```python
from build123d import *

# Parameters (mm, degrees)
SKETCH4_R           = 3.5
SKETCH4_R_2         = 19.25
BOSS_EXTRUDE1_DEPTH = 1
SKETCH5_R           = 19.25
BOSS_EXTRUDE2_DEPTH = 5
SKETCH6_R           = 18.5
BOSS_EXTRUDE3_DEPTH = 2
CUT_EXTRUDE1_DEPTH  = 6
SKETCH8_W           = 1
SKETCH8_H           = 25
CUT_EXTRUDE2_DEPTH  = 6
BOSS_EXTRUDE4_START = 4
SKETCH9_W           = 20
SKETCH9_H           = 18
BOSS_EXTRUDE4_DEPTH = 4
SKETCH10_R          = 4
BOSS_EXTRUDE5_DEPTH = 22
SKETCH11_R          = 3.5
BOSS_EXTRUDE6_DEPTH = 4
SKETCH12_R          = 2.75
CUT_EXTRUDE3_DEPTH  = 2
SKETCH13_R          = 1.5
CUT_EXTRUDE4_DEPTH  = 7
SKETCH14_W          = 35.5
SKETCH14_H          = 26
BOSS_EXTRUDE7_DEPTH = 20
BOSS_EXTRUDE8_DEPTH = 9.5
SKETCH16_W          = 15.5
SKETCH16_H          = 5
CUT_EXTRUDE5_DEPTH  = 8.5
SKETCH17_R          = 2
CUT_EXTRUDE6_DEPTH  = 4


with BuildPart() as part:
    # Sketch4 → Boss-Extrude1 (new body)
    with BuildSketch(Plane(origin=(0, 0, 0), x_dir=(1, 0, 0), z_dir=(0, 1, 0))):
        with Locations((-17.75, -21.25)):
            Circle(SKETCH4_R)
        with BuildLine():
            ThreePointArc((3e-08, -19.25), (-13.611805493, -13.611805583), (-19.25, -9.7e-08))
            Line((-19.25, -9.7e-08), (-19.25, -13))
            Line((-19.25, -13), (-21.140562134, -20.381617358))
            ThreePointArc((-21.140562134, -20.381617358), (-17.312374287, -17.777467245), (-14.25, -21.25))
            ThreePointArc((-14.25, -21.25), (-14.66103595, -22.895691677), (-15.797600627, -24.154847102))
            Line((-15.797600627, -24.154847102), (-8.5, -19.25))
            Line((-8.5, -19.25), (3e-08, -19.25))
        make_face()
        Circle(SKETCH4_R_2)
        with BuildLine():
            Line((19.25, -13), (19.25, 0))
            ThreePointArc((19.25, 0), (13.611805548, -13.611805527), (3e-08, -19.25))
            Line((3e-08, -19.25), (8.5, -19.25))
            Line((8.5, -19.25), (15.797600627, -24.154847102))
            ThreePointArc((15.797600627, -24.154847102), (15.7309919, -18.391048043), (21.140562134, -20.381617358))
            Line((21.140562134, -20.381617358), (19.25, -13))
        make_face()
        with Locations((17.75, -21.25)):
            Circle(SKETCH4_R)
        with BuildLine():
            Line((8.5, 19.25), (0, 19.25))
            ThreePointArc((0, 19.25), (13.611805538, 13.611805538), (19.25, 0))
            Line((19.25, 0), (19.25, 13))
            Line((19.25, 13), (21.140562134, 20.381617358))
            ThreePointArc((21.140562134, 20.381617358), (15.7309919, 18.391048043), (15.797600627, 24.154847102))
            Line((15.797600627, 24.154847102), (8.5, 19.25))
        make_face()
        with Locations((17.75, 21.25)):
            Circle(SKETCH4_R)
        with BuildLine():
            Line((-8.5, 19.25), (-15.797600627, 24.154847102))
            ThreePointArc((-15.797600627, 24.154847102), (-14.66103595, 22.895691677), (-14.25, 21.25))
            ThreePointArc((-14.25, 21.25), (-17.312374287, 17.777467245), (-21.140562134, 20.381617358))
            Line((-21.140562134, 20.381617358), (-19.25, 13))
            Line((-19.25, 13), (-19.25, -9.7e-08))
            ThreePointArc((-19.25, -9.7e-08), (-13.611805572, 13.611805504), (0, 19.25))
            Line((0, 19.25), (-8.5, 19.25))
        make_face()
        with Locations((-17.75, 21.25)):
            Circle(SKETCH4_R)
    extrude(amount=BOSS_EXTRUDE1_DEPTH)

    # Sketch5 → Boss-Extrude2 (add)
    with BuildSketch(Plane(origin=(0, 1, 0), x_dir=(1, 0, 0), z_dir=(0, 1, 0))):
        with Locations(Location((0, 0, 0), (0, 0, 270))):
            Circle(SKETCH5_R)
    extrude(amount=BOSS_EXTRUDE2_DEPTH)

    # Sketch6 → Boss-Extrude3 (add)
    with BuildSketch(Plane(origin=(0, 6, 0), x_dir=(1, 0, 0), z_dir=(0, 1, 0))):
        with Locations(Location((0, 0, 0), (0, 0, 270))):
            Circle(SKETCH6_R)
    extrude(amount=BOSS_EXTRUDE3_DEPTH)

    # Sketch7 → Cut-Extrude1 (cut)
    with BuildSketch(Plane(origin=(0, 8, 0), x_dir=(1, 0, 0), z_dir=(0, 1, 0))):
        with BuildLine():
            Line((-11.5, 13), (11.5, 13))
            ThreePointArc((11.5, 13), (17.356554958, 0), (11.5, -13))
            Line((11.5, -13), (-11.5, -13))
            ThreePointArc((-11.5, -13), (-17.356554958, 0), (-11.5, 13))
        make_face()
    extrude(amount=-CUT_EXTRUDE1_DEPTH, mode=Mode.SUBTRACT)

    # Sketch8 → Cut-Extrude2 (cut)
    with BuildSketch(Plane(origin=(0, 2, 0), x_dir=(1, 0, 0), z_dir=(0, 1, 0))):
        with Locations((-11, 0)):
            Rectangle(SKETCH8_W, SKETCH8_H)
        with Locations((11, 0)):
            Rectangle(SKETCH8_W, SKETCH8_H)
    extrude(amount=-CUT_EXTRUDE2_DEPTH, mode=Mode.SUBTRACT)

    # Sketch9 → Boss-Extrude4 (add)
    with BuildSketch(Plane(origin=(0, 2, 0), x_dir=(1, 0, 0), z_dir=(0, 1, 0)).offset(BOSS_EXTRUDE4_START)):
        Rectangle(SKETCH9_W, SKETCH9_H)
        with BuildLine():
            Line((-14.84082208, 9), (-12, 9))
            Line((-12, 9), (-12, -9))
            Line((-12, -9), (-14.84082208, -9))
            ThreePointArc((-14.84082208, -9), (-17.356554958, 0), (-14.84082208, 9))
        make_face()
        with BuildLine():
            Line((12, -9), (14.84082208, -9))
            ThreePointArc((14.84082208, -9), (17.356554958, 0), (14.84082208, 9))
            Line((14.84082208, 9), (12, 9))
            Line((12, 9), (12, -9))
        make_face()
    extrude(amount=-BOSS_EXTRUDE4_DEPTH)

    # Sketch10 → Boss-Extrude5 (add)
    with BuildSketch(Plane(origin=(0, 6, 0), x_dir=(1, 0, 0), z_dir=(0, 1, 0))):
        with Locations(Location((0, 0, 0), (0, 0, 270))):
            Circle(SKETCH10_R)
    extrude(amount=BOSS_EXTRUDE5_DEPTH)

    # Sketch11 → Boss-Extrude6 (add)
    with BuildSketch(Plane(origin=(0, 1, 0), x_dir=(1, 0, 0), z_dir=(0, 1, 0))):
        with Locations(Location((-17.75, 21.25, 0), (0, 0, 56.094250748))):
            Circle(SKETCH11_R)
        with Locations(Location((17.75, 21.25, 0), (0, 0, 123.905749252))):
            Circle(SKETCH11_R)
        with Locations(Location((17.75, -21.25, 0), (0, 0, 14.365660019))):
            Circle(SKETCH11_R)
        with Locations(Location((-17.75, -21.25, 0), (0, 0, 165.634339981))):
            Circle(SKETCH11_R)
    extrude(amount=BOSS_EXTRUDE6_DEPTH)

    # Sketch12 → Cut-Extrude3 (cut)
    with BuildSketch(Plane(origin=(0, 5, 0), x_dir=(1, 0, 0), z_dir=(0, 1, 0))):
        with Locations(Location((-17.75, 21.25, 0), (0, 0, 270))):
            Circle(SKETCH12_R)
        with Locations(Location((17.75, 21.25, 0), (0, 0, 270))):
            Circle(SKETCH12_R)
        with Locations(Location((17.75, -21.25, 0), (0, 0, 270))):
            Circle(SKETCH12_R)
        with Locations(Location((-17.75, -21.25, 0), (0, 0, 270))):
            Circle(SKETCH12_R)
    extrude(amount=-CUT_EXTRUDE3_DEPTH, mode=Mode.SUBTRACT)

    # Sketch13 → Cut-Extrude4 (cut)
    with BuildSketch(Plane(origin=(0, 3, 0), x_dir=(1, 0, 0), z_dir=(0, 1, 0))):
        with Locations(Location((-17.75, 21.25, 0), (0, 0, 270))):
            Circle(SKETCH13_R)
        with Locations(Location((17.75, 21.25, 0), (0, 0, 270))):
            Circle(SKETCH13_R)
        with Locations(Location((17.75, -21.25, 0), (0, 0, 270))):
            Circle(SKETCH13_R)
        with Locations(Location((-17.75, -21.25, 0), (0, 0, 270))):
            Circle(SKETCH13_R)
    extrude(amount=-CUT_EXTRUDE4_DEPTH, mode=Mode.SUBTRACT)

    # Sketch14 → Boss-Extrude7 (add)
    with BuildSketch(Plane.XZ):
        with Locations((0.5, 0)):
            Rectangle(SKETCH14_W, SKETCH14_H)
    extrude(amount=BOSS_EXTRUDE7_DEPTH)

    # Sketch15 → Boss-Extrude8 (add)
    with BuildSketch(Plane(origin=(18.25, 0, 0), x_dir=(0, 0, -1), z_dir=(1, 0, 0))):
        Polygon((-7.75, 0), (-7.75, -16), (7.75, -16), (7.75, 0), (7.75, 1), (-7.75, 1), align=None)
    extrude(amount=BOSS_EXTRUDE8_DEPTH)

    # Sketch16 → Cut-Extrude5 (cut)
    with BuildSketch(Plane(origin=(27.75, 0, 0), x_dir=(0, 0, -1), z_dir=(1, 0, 0))):
        with Locations((0, -1.5)):
            Rectangle(SKETCH16_W, SKETCH16_H)
    extrude(amount=-CUT_EXTRUDE5_DEPTH, mode=Mode.SUBTRACT)

    # Sketch17 → Cut-Extrude6 (cut)
    with BuildSketch(Plane.XZ):
        with Locations(Location((-17.75, 21.25, 0), (0, 0, 270))):
            Circle(SKETCH17_R)
        with Locations(Location((17.75, 21.25, 0), (0, 0, 270))):
            Circle(SKETCH17_R)
        with Locations(Location((17.75, -21.25, 0), (0, 0, 270))):
            Circle(SKETCH17_R)
        with Locations(Location((-17.75, -21.25, 0), (0, 0, 270))):
            Circle(SKETCH17_R)
    extrude(amount=-CUT_EXTRUDE6_DEPTH, mode=Mode.SUBTRACT)


solid = part.part
```
For this review, take the finished solid that the model builds, in its own axes (mm). A direction names the side the tool comes from. Coordinates: 2 decimals unless noted, no trailing zeros. Write each loop counter-clockwise with the first axis right and the second up, starting at its lowest first coordinate (ties: lowest second). Pieces come first, ordered by that corner, then holes. Notation, with made-up numbers: (71, 86.5) - (87, 86.5) arc R29 cw to (87, 121.5) - close; hole circle Ø2 at (-21, 73). An arc over 180 degrees is marked (long way). Answer in a Markdown table with one row per item. Add a question column.
Q1. We need section C-C, the plane y = -10. State the section outline as (x, z) points, and give its area (3 significant figures).
Q2. Tool access review of faces 4 (the flat face through (16, 3, 20)), 5 (the flat face through (23, -10, 7.75)), 6 (the flat face through (20.182, 0.493, -16.639)), 7 (the flat face through (0, -10, -13)): name each direction out of +Z, -Z, +X, -X, +Y, -Y from which nothing blocks a thin tool from reaching the whole face with its end or side.
Q3. We need section B-B, the plane z = 21.25. State the section outline as (x, y) points.
Q4. We need section D-D, the plane x = -2. State the section outline as (y, z) points, and give its area (3 significant figures).
Q5. For probe 1 along X at (y, z) = (3.55, 21.25); probe 2 along X at (y, z) = (2.1, -21.25); probe 3 along Z at (x, y) = (0.5, 3), list the stretches that pass through material, from the lowest coordinate up.
Q6. We need section A-A, the plane y = 4. Count the separate pieces of the cut face and the enclosed holes in it, and give its area (3 significant figures).
Q7. For P1, Ø3, axis at y = 5, z = 0.5, coming from the +X side; P2, Ø6, axis at y = 8.5, z = -14.5, coming from the +X side; P3, Ø5, axis at x = 17.75, z = 21.25, coming from the -Y side, all flat-tipped, find the tip position at first contact; note any pin that passes through.
Q8. Draft analysis for pull direction X (two halves, no side actions). For faces 1 (the flat face through (0, 5, -13)), 2 (the flat face through (23, -16, 0)), 3 (the flat face through (27.75, -10, 0)), state which applies: +X half, -X half, draft (parallel to the pull), parting line (faces both ways), or undercut.
Answer list:
| question | item | result |
|---|---|---|
| 1 | outline | (-17.25, -13) - (18.25, -13) - (18.25, -7.75) - (27.75, -7.75) - (27.75, 7.75) - (18.25, 7.75) - (18.25, 13) - (-17.25, 13) - close |
| 1 | area | 1,070 mm2 |
| 2 | face 4 | +Y |
| 2 | face 5 | +Z, +X, -Y |
| 2 | face 6 | +X, +Y, -Y |
| 2 | face 7 | -Z, +X, -X, -Y |
| 3 | outline | (-21.25, 0) - (-19.75, 0) - (-19.75, 3) - (-20.5, 3) - (-20.5, 5) - (-21.25, 5) - close; (-15.75, 0) - (-11.48, 0) - (-11.48, 1) - (-14.25, 1) - (-14.25, 5) - (-15, 5) - (-15, 3) - (-15.75, 3) - close; (11.48, 0) - (15.75, 0) - (15.75, 3) - (15, 3) - (15, 5) - (14.25, 5) - (14.25, 1) - (11.48, 1) - close; (19.75, 0) - (21.25, 0) - (21.25, 5) - (20.5, 5) - (20.5, 3) - (19.75, 3) - close |
| 4 | outline | (-20, -13) - (0, -13) - (0, -19.25) - (1, -19.25) - (1, -19.15) - (6, -19.15) - (6, -18.39) - (8, -18.39) - (8, -13) - (2, -13) - (2, -9) - (6, -9) - (6, -3.46) - (28, -3.46) - (28, 3.46) - (6, 3.46) - (6, 9) - (2, 9) - (2, 13) - (8, 13) - (8, 18.39) - (6, 18.39) - (6, 19.15) - (1, 19.15) - (1, 19.25) - (0, 19.25) - (0, 13) - (-20, 13) - close |
| 4 | area | 892 mm2 |
| 5 | probe 1 | x = -21.25 to -20.5, -15 to -14.25, 14.25 to 15, 20.5 to 21.25 |
| 5 | probe 2 | x = -21.25 to -19.75, -15.75 to -14.25, 14.25 to 15.75, 19.75 to 21.25 |
| 5 | probe 3 | z = -19.24 to -13, -9 to 9, 13 to 19.24 |
| 6 | separate pieces | 6 |
| 6 | enclosed holes | 5 |
| 6 | area | 938 mm2 |
| 7 | P1 | stops at x = 19.25 |
| 7 | P2 | stops at x = 14.46 |
| 7 | P3 | stops at y = 0 |
| 8 | face 1 | undercut |
| 8 | face 2 | draft |
| 8 | face 3 | +X half |
